```python
from build123d import *

# Parameters (mm, degrees)
SKETCH1_R           = 7.5
BOSS_EXTRUDE1_DEPTH = 30
SKETCH2_W           = 20
SKETCH2_H           = 4
CUT_EXTRUDE1_DEPTH  = 15
SKETCH3_R           = 2.5
CUT_EXTRUDE2_DEPTH  = 7.5
SKETCH4_R           = 12.5
BOSS_EXTRUDE2_DEPTH = 15


with BuildPart() as part:
    # Sketch1 → Boss-Extrude1 (new, symmetric)
    with BuildSketch(Plane.XY):
        Circle(SKETCH1_R)
    extrude(amount=BOSS_EXTRUDE1_DEPTH, both=True)

    # Sketch2 → Cut-Extrude1 (cut)
    with BuildSketch(Plane.XY.offset(30)):
        Rectangle(SKETCH2_W, SKETCH2_H)
    extrude(amount=-CUT_EXTRUDE1_DEPTH, mode=Mode.SUBTRACT)

    # Sketch3 → Cut-Extrude2 (cut, symmetric)
    with BuildSketch(Plane(origin=(0, 0, 0), x_dir=(1, 0, 0), z_dir=(0, 1, 0))):
        with Locations(Location((0, -23, 0), (0, 0, 270))):
            Circle(SKETCH3_R)
    extrude(amount=CUT_EXTRUDE2_DEPTH, both=True, mode=Mode.SUBTRACT)

    # Sketch4 → Boss-Extrude2 (add)
    with BuildSketch(Plane(origin=(0, 0, -30), x_dir=(-1, 0, 0), z_dir=(0, 0, -1))):
        Circle(SKETCH4_R)
    extrude(amount=-BOSS_EXTRUDE2_DEPTH)


solid = part.part
```
The listing builds one solid part. Answer for the finished solid, in the listing's coordinates (mm). A direction names the side the tool comes from. Give positions to 0.01 mm unless a question says otherwise; leave off trailing zeros. Order: outer loops, then holes, each group sorted by start corner. A loop starts at its lowest first (then second) coordinate and runs counter-clockwise, first axis right, second up. Notation, with made-up numbers: (15.25, -14) - (19.25, -14) arc R19 cw to (19.25, -8) - close; hole circle Ø9 at (14.25, -12). An arc over 180 degrees is marked (long way). Use one line per item in the form item = value. Start each with the question number.
(1) A cutting plane is placed at C-C, the plane z = 23. Write down the section's boundary in (x, y), then the cut area to 3 significant figures.
(2) A cutting plane is placed at B-B, the plane y = 0. Write down the section's boundary in (x, z), then the cut area to 3 significant figures.
(3) Flat-ended cylindrical pins translate along their axes: pin 1 Ø2 at (y, z) = (-2, -16.5) entering from -X; pin 2 Ø5 at (x, z) = (-5, 7) entering from -Y; pin 3 Ø7 at (x, z) = (2, 21.5) entering from -Y. Find the tip coordinate at first contact, or state that the pin passes through.
(4) For faces 5 (the cylindrical face through (6.93, -2.87, 7.82)), 6 (the flat face through (-2, -2, 21)), 7 (the flat face through (0, -4, 30)), determine the directions among +Z, -Z, +X, -X, +Y, -Y from which every point of the face is accessible in a straight line to the end or side of a thin tool.
(5) The mould has two halves that part along Y. Classify faces 1 (the flat face through (0, 0, 15)), 2 (the flat face through (0, -8, -15)), 3 (the cylindrical face through (-11.923, 3.755, -22.605)), 4 (the flat face through (-2, 2, 21)): released by +Y, released by -Y, zero draft, split by the parting line, or undercut.
(6) A cutting plane is placed at A-A, the plane x = 0. Write down the section's boundary in (y, z), then the cut area to 3 significant figures.
(7) A cutting plane is placed at D-D, the plane y = 5.5. Write down the section's boundary in (x, z), then the cut area to 3 significant figures.
(8) Consider line 1 (Z direction, x = 0, y = 5.8); line 2 (Z direction, x = -10.5, y = 4.75); line 3 (X direction, y = -5.6, z = 23). Determine where each line is inside the solid, lowest interval first. Write a range as from..to.
Ans:
q1.outline = (-7.23, -2) arc R7.5 ccw to (-2.5, -7.07) - (-2.5, -2) - close; (-7.23, 2) - (-2.5, 2) - (-2.5, 7.07) arc R7.5 ccw to start; (2.5, -7.07) arc R7.5 ccw to (7.23, -2) - (2.5, -2) - close; (2.5, 2) - (7.23, 2) arc R7.5 ccw to (2.5, 7.07) - close
q1.area = 63.8 mm^2
q2.outline = (-12.5, -30) - (12.5, -30) - (12.5, -15) - (7.5, -15) - (7.5, 15) - (-7.5, 15) - (-7.5, -15) - (-12.5, -15) - close
q2.area = 825 mm^2
q3.pin_1 = -12.46
q3.pin_2 = -7.07
q3.pin_3 = -7.5
q4.face_5 = +Z
q4.face_6 = +Z, +X, -X
q4.face_7 = +Z, +X, -X, +Y, -Y
q5.face_1 = undercut
q5.face_2 = zero draft
q5.face_3 = split by the parting line
q5.face_4 = undercut
q6.outline = (-12.5, -30) - (12.5, -30) - (12.5, -15) - (7.5, -15) - (7.5, 20.5) - (2, 20.5) - (2, 15) - (-2, 15) - (-2, 20.5) - (-7.5, 20.5) - (-7.5, -15) - (-12.5, -15) - close; (-7.5, 25.5) - (-2, 25.5) - (-2, 30) - (-7.5, 30) - close; (2, 25.5) - (7.5, 25.5) - (7.5, 30) - (2, 30) - close
q6.area = 935 mm^2
q7.outline = (-11.22, -30) - (11.22, -30) - (11.22, -15) - (5.1, -15) - (5.1, 30) - (-5.1, 30) - (-5.1, -15) - (-11.22, -15) - close; hole circle Ø5 at (0, 23)
q7.area = 776 mm^2
q8.line_1 = -30..20.5, 25.5..30
q8.line_2 = -30..-15
q8.line_3 = -4.99..-2.5, 2.5..4.99
